The listing builds one solid part. Answer for the finished solid, in the listing's coordinates (mm). A direction names the side the tool comes from. Coordinates: 2 decimals unless noted, no trailing zeros. Loops run counter-clockwise (first coordinate to the right, second up) from the corner with the lowest first, then second, coordinate; pieces in that order, holes last. Notation, with made-up numbers: (89.25, -38.5) - (145.25, -38.5) arc R22 cw to (145.25, -4.5) - close; hole circle Ø1 at (21, -28). An arc over 180 degrees is marked (long way). One line per question, with ' | ' between items.
from build123d import *

# Parameters (mm, degrees)
F0_W     = 50
F0_H     = 50
F0_W_2   = 40
F0_H_2   = 40
F1_DEPTH = 25
F2_W     = 50
F2_H     = 50
F2_W_2   = 40
F2_H_2   = 40
F3_DEPTH = 25
F4_SIZE  = 24.99999


# Not quite as in the source:
# - a fillet or chamfer is up to 0.001 mm smaller than in the source, because OpenCascade refuses the exact size


with BuildPart() as f1:
    # F0 (on Top) → F1 (new body)
    with BuildSketch(Plane.XY):
        with Locations((25, 25)):
            Rectangle(F0_W, F0_H)
        with Locations((25, 25)):
            Rectangle(F0_W_2, F0_H_2, mode=Mode.SUBTRACT)
    extrude(amount=F1_DEPTH)

    # F2 (on face) → F3 (join)
    with BuildSketch(Plane.XY.offset(25)):
        with Locations((25, 25)):
            Rectangle(F2_W, F2_H)
        with Locations((25, 25)):
            Rectangle(F2_W_2, F2_H_2, mode=Mode.SUBTRACT)
        with Locations((25, 25)):
            Rectangle(F2_W_2, F2_H_2)
    extrude(amount=F3_DEPTH)

    # F4 (size 25 in the source; OpenCascade refuses exactly that, so slightly less here)
    f4_edges = [f1.edges().sort_by_distance(p)[0] for p in [
        (25, 0, 50),
        (25, 50, 50),
    ]]
    chamfer(f4_edges, length=F4_SIZE)


solid = f1.part
Item 1: Find section A-A, the plane z = 20. Write down the section's boundary in (x, y).
Taken from the geometry:
outline: (0, 0) - (50, 0) - (50, 50) - (0, 50) - close; hole (5, 5) - (45, 5) - (45, 45) - (5, 45) - close
Item 2: The mould has two halves that part along Y. Classify faces 1 (the face through (50, 25, 19)), 2 (the face through (25, 5, 12)), 3 (the face through (25, 25, 25)), 4 (the face through (25, 13, 38)): pulls with the +Y half, pulls with the -Y half, needs draft (parallel to the pull), parting line crosses it, or undercut.
Taken from the geometry:
face 1: needs draft | face 2: undercut | face 3: undercut | face 4: pulls with the -Y half
Item 3: Find the intervals of material crossed by line 1 (Y direction, x = 44.5, z = 12); line 2 (Z direction, x = 42.5, y = 47), in increasing order. Write a range as [from, to].
Taken from the geometry:
line 1: y = [0, 5], [45, 50] | line 2: z = [0, 28]
Item 4: Each of these flat-tipped pins is pushed along its axis until it touches: pin 1 Ø12 at (x, y) = (16.5, 27) entering from -Z; pin 2 Ø1 at (x, y) = (39, 40.5) entering from +Z; pin 3 Ø5 at (x, y) = (28, 36) entering from +Z. Where does it stop, or does it pass through?
Taken from the geometry:
pin 1: stops at z = 25 | pin 2: stops at z = 35 | pin 3: stops at z = 41.5
Item 5: Find section C-C, the plane y = 20.5. Write down the section's boundary in (x, z).
Taken from the geometry:
outline: (0, 0) - (5, 0) - (5, 25) - (45, 25) - (45, 0) - (50, 0) - (50, 45.5) - (0, 45.5) - close
Item 6: Which of the six approach directions +Z, -Z, +X, -X, +Y, -Y give full straight-line access (tool end or side, diameter ignored) to faces 5 (the face through (0, 25, 19)), 6 (the face through (45, 25, 12))?
Taken from the geometry:
face 5: +Z, -Z, -X, +Y, -Y | face 6: -Z
